Read the model definition and answer for the solid it produces. Units are mm, in the model's axes. A direction names the side the tool comes from. Coordinates: 2 decimals unless noted, no trailing zeros. Loops run counter-clockwise (first coordinate to the right, second up) from the corner with the lowest first, then second, coordinate; pieces in that order, holes last. Notation, with made-up numbers: M 29,89.25 L 46,89.25 A15 ccw 46,102.25 Z; hole C 83,19 d6. An arc over 180 degrees is marked long. One line per item, written item: value. Start each with the question number.
1. Consider probe 1 along X at (y, z) = (1.2, -56.75); probe 2 along X at (y, z) = (3.35, -26.5); probe 3 along X at (y, z) = (5.2, -6.5). Determine where each line is inside the solid, lowest interval first.
2. Determine the mould class of faces 1 (the face through (25, 3, -6)), 2 (the face through (92, 3, -37)), 3 (the face through (6, 3, -15)) for opening direction Z: +Z half, -Z half, draft (parallel to the pull), parting line (faces both ways), or undercut.
3. The part is cut by section D-D (z = -22). Write down the section's boundary in (x, y).
4. The part is cut by section A-A (x = 77.75). Write down the section's boundary in (y, z).
5. For faces 4 (the face through (94, 3, -25)), 5 (the face through (43, 3, -72)), 6 (the face through (124, 3, -60)), determine the directions among +Z, -Z, +X, -X, +Y, -Y from which every point of the face is accessible in a straight line to the end or side of a thin tool.
6. The part is cut by section C-C (y = 5.1). State how many separate pieces and enclosed holes the cut face has, then the cut area to 3 significant figures.
7. The part is cut by section B-B (z = -56.75). Write down the section's boundary in (x, y).
8. Flat-ended cylindrical pins translate along their axes: pin 1 (3 mm diameter, centred on x = 29, y = 3.5, fed in from +Z); pin 2 (3 mm diameter, centred on x = 126, y = 3, fed in from -Z); pin 3 (2 mm diameter, centred on y = 3, z = -22, fed in from +X). Find the tip coordinate at first contact, or state that the pin passes through.
```python
from build123d import *

# Parameters (mm, degrees)
SKETCH1_W           = 130
SKETCH1_H           = 75
BOSS_EXTRUDE1_DEPTH = 6
SKETCH2_R           = 8
CUT_EXTRUDE1_DEPTH  = 6
SKETCH3_W           = 4
SKETCH3_H           = 25
CUT_EXTRUDE2_DEPTH  = 151.203195705


with BuildPart() as part:
    # Sketch1 → Boss-Extrude1 (new body)
    with BuildSketch(Plane(origin=(0, 0, 0), x_dir=(1, 0, 0), z_dir=(0, 1, 0))):
        with Locations((65, 37.5)):
            Rectangle(SKETCH1_W, SKETCH1_H)
    extrude(amount=BOSS_EXTRUDE1_DEPTH)

    # Sketch2 → Cut-Extrude1 (cut)
    with BuildSketch(Plane(origin=(0, 6, 0), x_dir=(1, 0, 0), z_dir=(0, 1, 0))):
        with Locations(Location((52.25, 56.75, 0), (0, 0, 270))):
            Circle(SKETCH2_R)
        with Locations(Location((77.75, 56.75, 0), (0, 0, 270))):
            Circle(SKETCH2_R)
    extrude(amount=-CUT_EXTRUDE1_DEPTH, mode=Mode.SUBTRACT)

    # Sketch3 → Cut-Extrude2 (cut, through all)
    with BuildSketch(Plane(origin=(0, 6, 0), x_dir=(1, 0, 0), z_dir=(0, 1, 0))):
        Polygon((0, 0), (43, 0), (43, 6), (6, 6), (6, 25), (0, 25), align=None)
        Polygon((0, 50), (6, 50), (6, 69), (43, 69), (43, 75), (0, 75), align=None)
        with Locations((36, 37.5)):
            Rectangle(SKETCH3_W, SKETCH3_H)
        Polygon((87, 6), (87, 0), (130, 0), (130, 25), (124, 25), (124, 6), align=None)
        with Locations((94, 37.5)):
            Rectangle(SKETCH3_W, SKETCH3_H)
        Polygon((87, 75), (87, 69), (124, 69), (124, 50), (130, 50), (130, 75), align=None)
    extrude(amount=-CUT_EXTRUDE2_DEPTH, mode=Mode.SUBTRACT)


solid = part.part
```
Answer block:
1. probe 1: x = 6 to 44.25, 60.25 to 69.75, 85.75 to 124
1. probe 2: x = 0 to 34, 38 to 92, 96 to 130
1. probe 3: x = 6 to 124
2. face 1: +Z half
2. face 2: undercut
2. face 3: draft
3. outline: M 6,0 L 124,0 L 124,6 L 6,6 Z
4. outline: M 0,-75 L 6,-75 L 6,-64.75 L 0,-64.75 Z; M 0,-48.75 L 6,-48.75 L 6,0 L 0,0 Z
5. face 4: +Y, -Y
5. face 5: -Z, -X, +Y, -Y
5. face 6: -Z, +X, +Y, -Y
6. separate pieces: 1
6. enclosed holes: 4
6. area: 7,660 mm2
7. outline: M 6,0 L 44.25,0 L 44.25,6 L 6,6 Z; M 60.25,0 L 69.75,0 L 69.75,6 L 60.25,6 Z; M 85.75,0 L 124,0 L 124,6 L 85.75,6 Z
8. pin 1: stops at z = -6
8. pin 2: stops at z = -50
8. pin 3: stops at x = 124
